For this review, take the finished solid that the model builds, in its own axes (mm). Face numbers are marked on the shaded views. A direction names the side the tool comes from. Round coordinates to 2 decimals unless told otherwise and drop trailing zeros. Write each loop counter-clockwise with the first axis right and the second up, starting at its lowest first coordinate (ties: lowest second). Pieces come first, ordered by that corner, then holes. Notation, with made-up numbers: (24, -1) - (79, -1) arc R12 ccw to (79, 21) - close; hole circle Ø1 at (11.5, -24). An arc over 180 degrees is marked (long way). One line per item, written item: value. Start each with the question number.
Q1. Add section A-A on y = -2. Write out the cut boundary in (x, z).
Q2. Clearance check with flat-ended pins moving along their axes: pin 1 Ø0.6 at (y, z) = (-2.5, 0.5) entering from +X; pin 2 Ø4 at (x, z) = (-3.5, 0) entering from +Y; pin 3 Ø2 at (x, y) = (0, -3.5) entering from +Z. State where each tip first meets the part, or that it passes through.
Q3. Add section B-B on x = 0. Write out the cut boundary in (y, z).
Q4. For probe 1 along Y at (x, z) = (0, 6.1); probe 2 along Z at (x, y) = (-0.75, -5.25); probe 3 along Y at (x, z) = (-4.25, 2.5), list the stretches that pass through material, from the lowest coordinate up.
Q5. Add section D-D on z = 0.75. Write out the cut boundary in (x, y), and give its area (3 significant figures).
Q6. Tool access review of the marked faces 1, 2 and 3: name each direction out of +Z, -Z, +X, -X, +Y, -Y from which nothing blocks a thin tool from reaching the whole face with its end or side.
Q7. Mouldability with a two-part tool opening along X and no side actions: class the marked faces 4, 5, 6 and 7 as +X half, -X half, draft (parallel to the pull), parting line (faces both ways), or undercut.
Q8. Add section C-C on y = -0.5. Write out the cut boundary in (x, z).
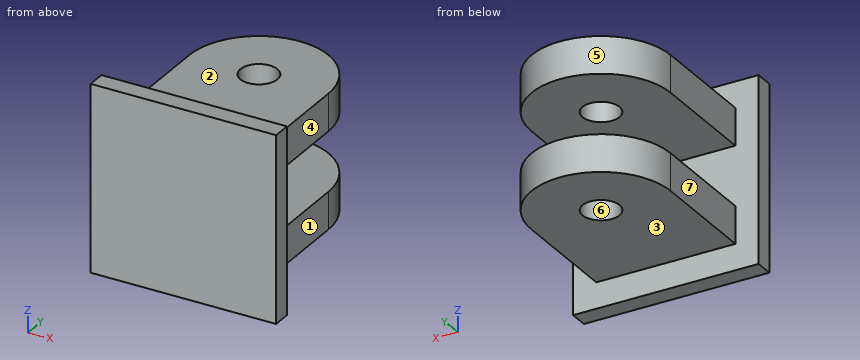
```python
from build123d import *

# Parameters (mm, degrees)
CROQUIS1_R              = 1
SALIENTE_EXTRUIR1_DEPTH = 2
MATRIZL1_COUNT          = 2
MATRIZL1_PITCH          = 5.2
CROQUIS2_W              = 10
CROQUIS2_H              = 10
SALIENTE_EXTRUIR2_DEPTH = 1


with BuildPart() as part:
    # Croquis1 → Saliente-Extruir1 (new body)
    with BuildSketch(Plane.XY):
        with BuildLine():
            Line((-3.75, 0), (-3.75, -6))
            Line((-3.75, -6), (3.75, -6))
            Line((3.75, -6), (3.75, 0))
            ThreePointArc((3.75, 0), (0, 3.75), (-3.75, 0))
        make_face()
        Circle(CROQUIS1_R, mode=Mode.SUBTRACT)
    extrude(amount=SALIENTE_EXTRUIR1_DEPTH)


with BuildPart() as matrizl1_1:
    # MatrizL1: pattern copy
    add(part.part.moved(Location(Vector(0, 0, 1) * (1 * MATRIZL1_PITCH))))


with BuildPart() as part_1:
    add(part.part)

    add(matrizl1_1.part)  # Saliente-Extruir2 merges MatrizL1_1
    # Croquis2 → Saliente-Extruir2 (add)
    with BuildSketch(Plane.XZ.offset(6)):
        with Locations((0, 3.6)):
            Rectangle(CROQUIS2_W, CROQUIS2_H)
    extrude(amount=SALIENTE_EXTRUIR2_DEPTH)


solid = part_1.part
```
Result set:
1. outline: (-3.75, 0) - (3.75, 0) - (3.75, 2) - (-3.75, 2) - close; (-3.75, 5.2) - (3.75, 5.2) - (3.75, 7.2) - (-3.75, 7.2) - close
2. pin 1: stops at x = 3.75
2. pin 2: stops at y = 3.44
2. pin 3: stops at z = 7.2
3. outline: (-7, -1.4) - (-6, -1.4) - (-6, 0) - (-1, 0) - (-1, 2) - (-6, 2) - (-6, 5.2) - (-1, 5.2) - (-1, 7.2) - (-6, 7.2) - (-6, 8.6) - (-7, 8.6) - close; (1, 0) - (3.75, 0) - (3.75, 2) - (1, 2) - close; (1, 5.2) - (3.75, 5.2) - (3.75, 7.2) - (1, 7.2) - close
4. probe 1: y = -7 to -1, 1 to 3.75
4. probe 2: z = 0 to 2, 5.2 to 7.2
4. probe 3: y = -7 to -6
5. outline: (-5, -7) - (5, -7) - (5, -6) - (3.75, -6) - (3.75, 0) arc R3.75 ccw to (-3.75, 0) - (-3.75, -6) - (-5, -6) - close; hole circle Ø2 at (0, 0)
5. area: 73.9 mm^2
6. face 1: +Z, -Z, +X, +Y
6. face 2: +Z, +X, -X, +Y
6. face 3: -Z, +X, -X, +Y
7. face 4: +X half
7. face 5: parting line
7. face 6: undercut
7. face 7: -X half
8. outline: (-3.75, 0) - (-0.87, 0) - (-0.87, 2) - (-3.75, 2) - close; (-3.75, 5.2) - (-0.87, 5.2) - (-0.87, 7.2) - (-3.75, 7.2) - close; (0.87, 0) - (3.75, 0) - (3.75, 2) - (0.87, 2) - close; (0.87, 5.2) - (3.75, 5.2) - (3.75, 7.2) - (0.87, 7.2) - close
